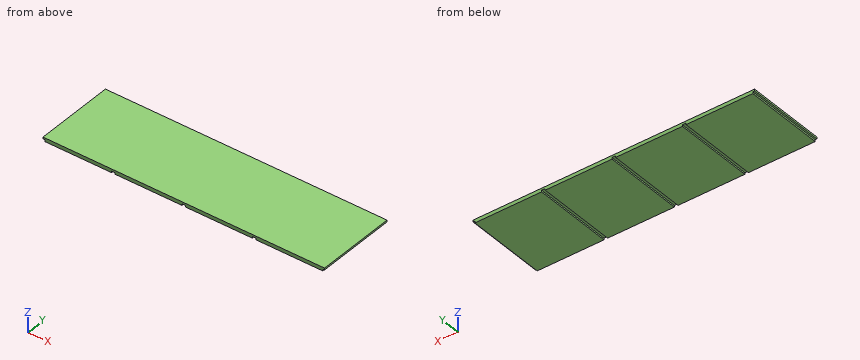
from build123d import *

# Parameters (mm, degrees)
SKETCH_W        = 1404
SKETCH_H        = 400
PAD_DEPTH       = 18
SKETCH001_W     = 9
SKETCH001_H     = 400
POCKET_DEPTH    = 9
SKETCH002_W     = 18
SKETCH002_H     = 400
POCKET001_DEPTH = 8


with BuildPart() as part:
    # Sketch → Pad (new body)
    with BuildSketch(Plane.XY):
        with Locations((-702, 200)):
            Rectangle(SKETCH_W, SKETCH_H)
    extrude(amount=PAD_DEPTH)

    # Sketch001 → Pocket (cut)
    with BuildSketch(Plane.XY):
        with Locations((-4.5, 200)):
            Rectangle(SKETCH001_W, SKETCH001_H)
        with Locations((-1399.5, 200)):
            Rectangle(SKETCH001_W, SKETCH001_H)
    extrude(amount=POCKET_DEPTH, mode=Mode.SUBTRACT)

    # Sketch002 (on Face4 of Pocket) → Pocket001 (cut)
    with BuildSketch(Plane(origin=(0, 0, 0), x_dir=(1, 0, 0), z_dir=(0, 0, -1))):
        with Locations((-351, -200)):
            Rectangle(SKETCH002_W, SKETCH002_H)
        with Locations((-702, -200)):
            Rectangle(SKETCH002_W, SKETCH002_H)
        with Locations((-1053, -200)):
            Rectangle(SKETCH002_W, SKETCH002_H)
    extrude(amount=-POCKET001_DEPTH, mode=Mode.SUBTRACT)


solid = part.part
Could you check a few things on this model? Use its own coordinates, in mm. Give positions to 0.01 mm unless a question says otherwise; leave off trailing zeros. Write each loop counter-clockwise with the first axis right and the second up, starting at its lowest first coordinate (ties: lowest second). Pieces come first, ordered by that corner, then holes. Notation, with made-up numbers: (-3, 1) -> (44, 1) arc R18 ccw to (44, 11) -> close; hole circle Ø5 at (-19.75, -6). An arc over 180 degrees is marked (long way). Answer as CSV lines item,"result". Start each with the question number.
(1) Please list where these lines run through material, in increasing order: line 1 (X direction, y = 298.5, z = 3.25); line 2 (X direction, y = 211.5, z = 8.25).
(2) If we section it at B-B, the plane y = 80: Write out the boundary of the cut face in (x, z).
(3) I'm going to push flat-ended pins straight in: pin 1 Ø2.5 at (y, z) = (264, 4.5) entering from -X; pin 2 Ø9 at (y, z) = (264, 2.5) entering from +X; pin 3 Ø2.5 at (x, y) = (-5, 134.5) entering from -Z. Where does each tip first touch, or does it pass through?
(4) If we section it at A-A, the plane z = 4.75: Write out the boundary of the cut face in (x, y), and give its area (3 significant figures).
Answer list:
1,line 1,"-1395 to -1062, -1044 to -711, -693 to -360, -342 to -9"
1,line 2,"-1395 to -9"
2,outline,"(-1404, 9) -> (-1395, 9) -> (-1395, 0) -> (-1062, 0) -> (-1062, 8) -> (-1044, 8) -> (-1044, 0) -> (-711, 0) -> (-711, 8) -> (-693, 8) -> (-693, 0) -> (-360, 0) -> (-360, 8) -> (-342, 8) -> (-342, 0) -> (-9, 0) -> (-9, 9) -> (0, 9) -> (0, 18) -> (-1404, 18) -> close"
3,pin 1,"x = -1395"
3,pin 2,"x = -9"
3,pin 3,"z = 9"
4,outline,"(-1395, 0) -> (-1062, 0) -> (-1062, 400) -> (-1395, 400) -> close; (-1044, 0) -> (-711, 0) -> (-711, 400) -> (-1044, 400) -> close; (-693, 0) -> (-360, 0) -> (-360, 400) -> (-693, 400) -> close; (-342, 0) -> (-9, 0) -> (-9, 400) -> (-342, 400) -> close"
4,area,"533,000 mm^2"
